The model under review builds one solid part; all positions refer to its coordinate system, in mm. Face numbers are marked on the shaded views. A direction names the side the tool comes from. Coordinates: 2 decimals unless noted, no trailing zeros. Write each loop counter-clockwise with the first axis right and the second up, starting at its lowest first coordinate (ties: lowest second). Pieces come first, ordered by that corner, then holes. Notation, with made-up numbers: M 74.5,71 L 98.5,71 A9 ccw 98.5,88 Z; hole C 36,63.5 d11. An arc over 180 degrees is marked long. Answer as a JSON object with one key per item and string values.
```python
from build123d import *

# Parameters (mm, degrees)
SKETCH2_W           = 56.399999976
SKETCH2_H           = 56.399999976
SKETCH2_R           = 15.8877
SKETCH2_R_2         = 2.499999953
BOSS_EXTRUDE1_DEPTH = 6.35
SKETCH2_4_R         = 19.05
SKETCH2_4_R_2       = 15.8877
CUT_EXTRUDE2_DEPTH  = 1.600000102
SKETCH3_R           = 25.4
SKETCH3_R_2         = 19.05
BOSS_EXTRUDE2_DEPTH = 47.625
SKETCH4_R           = 2.5
SKETCH4_R_2         = 7.62
BOSS_EXTRUDE3_DEPTH = 6.35
FILLET1_R           = 2.54


with BuildPart() as part:
    # Sketch2 → Boss-Extrude1 (new body)
    with BuildSketch(Plane(origin=(0, 0, 0), x_dir=(1, 0, 0), z_dir=(0, 1, 0))):
        Rectangle(SKETCH2_W, SKETCH2_H)
        with Locations(Location((0, 0, 0), (0, 0, 270))):
            Circle(SKETCH2_R, mode=Mode.SUBTRACT)
        with Locations(Location((23.569999977, 23.569999977, 0), (0, 0, 270))):
            Circle(SKETCH2_R_2, mode=Mode.SUBTRACT)
        with Locations(Location((23.569999977, -23.569999977, 0), (0, 0, 270))):
            Circle(SKETCH2_R_2, mode=Mode.SUBTRACT)
        with Locations(Location((-23.569999977, -23.569999977, 0), (0, 0, 270))):
            Circle(SKETCH2_R_2, mode=Mode.SUBTRACT)
        with Locations(Location((-23.569999977, 23.569999977, 0), (0, 0, 270))):
            Circle(SKETCH2_R_2, mode=Mode.SUBTRACT)
    extrude(amount=-BOSS_EXTRUDE1_DEPTH)

    # Sketch2<4> → Cut-Extrude2 (cut)
    with BuildSketch(Plane(origin=(0, 0, 0), x_dir=(1, 0, 0), z_dir=(0, 1, 0))):
        with Locations(Location((0, 0, 0), (0, 0, 270))):
            Circle(SKETCH2_4_R)
        with Locations(Location((0, 0, 0), (0, 0, 270))):
            Circle(SKETCH2_4_R_2, mode=Mode.SUBTRACT)
    extrude(amount=-CUT_EXTRUDE2_DEPTH, mode=Mode.SUBTRACT)

    # Sketch3 → Boss-Extrude2 (add)
    with BuildSketch(Plane.XZ.offset(6.35)):
        with Locations(Location((0, 0, 0), (0, 0, 270))):
            Circle(SKETCH3_R)
        with Locations(Location((0, 0, 0), (0, 0, 90))):
            Circle(SKETCH3_R_2, mode=Mode.SUBTRACT)
    extrude(amount=BOSS_EXTRUDE2_DEPTH)

    # Sketch4 → Boss-Extrude3 (add)
    with BuildSketch(Plane.XZ.offset(53.975)):
        with BuildLine():
            Line((38.1, -14.999999972), (38.1, 14.999999972))
            Line((38.1, 14.999999972), (20.497804781, 14.999999972))
            ThreePointArc((20.497804781, 14.999999972), (0, 25.4), (-20.497804781, 14.999999972))
            Line((-20.497804781, 14.999999972), (-38.1, 14.999999972))
            Line((-38.1, 14.999999972), (-38.1, -14.999999972))
            Line((-38.1, -14.999999972), (-20.497804781, -14.999999972))
            ThreePointArc((-20.497804781, -14.999999972), (0, -25.4), (20.497804781, -14.999999972))
            Line((20.497804781, -14.999999972), (38.1, -14.999999972))
        make_face()
        with Locations(Location((-33.655, -10.554999972, 0), (0, 0, 270))):
            Circle(SKETCH4_R, mode=Mode.SUBTRACT)
        with Locations(Location((0, 0, 0), (0, 0, 270))):
            Circle(SKETCH4_R_2, mode=Mode.SUBTRACT)
        with Locations(Location((-33.655, 10.554999972, 0), (0, 0, 270))):
            Circle(SKETCH4_R, mode=Mode.SUBTRACT)
        with Locations(Location((33.655, -10.554999972, 0), (0, 0, 270))):
            Circle(SKETCH4_R, mode=Mode.SUBTRACT)
        with Locations(Location((33.655, 10.554999972, 0), (0, 0, 270))):
            Circle(SKETCH4_R, mode=Mode.SUBTRACT)
    extrude(amount=BOSS_EXTRUDE3_DEPTH)

    # Fillet1
    # the kernel refuses this fillet: 2.54 mm, written as the material it adds along each edge
    with BuildSketch(Plane(origin=(20.497804781, -53.975, 14.999999972), x_dir=(-0.6093303633188096, 0, 0.7929164573508154), z_dir=(0, -1, 0)), Plane(origin=(-20.497804781, -53.975, -14.999999972), x_dir=(0.609330363318784, 0, -0.7929164573508352), z_dir=(0, -1, 0))) as fillet1_piece_1:
        with BuildLine():
            CenterArc((1.251994792, -2.539300218), FILLET1_R, 91.344968241, 51.113932151)
            Line((-0.762013009, -0.991601095), (0, 0))
            ThreePointArc((0, 0), (0.596187996, -0.006997817), (1.192375993, 0))
        make_face()
    extrude(amount=6.35)
    with BuildSketch(Plane(origin=(-20.497804781, -53.975, 14.999999972), x_dir=(0.6093303633187793, 0, 0.7929164573508387), z_dir=(0, -1, 0)), Plane(origin=(20.497804781, -53.975, -14.999999972), x_dir=(-0.609330363318815, 0, -0.7929164573508114), z_dir=(0, -1, 0))) as fillet1_piece_2:
        with BuildLine():
            CenterArc((1.251994792, 2.539300218), FILLET1_R, 217.541099608, 51.113932151)
            Line((-0.762013009, 0.991601095), (0, 0))
            ThreePointArc((0, 0), (0.596187996, 0.006997817), (1.192375993, 0))
        make_face()
    extrude(amount=6.35)
    # the kernel refuses this fillet: 2.54 mm, written as the material it takes off along each edge
    with BuildSketch(Plane(origin=(-28.199999988, 6.35, -28.199999988), x_dir=(0, 0, 1), z_dir=(0, -1, 0)), Plane(origin=(-28.199999988, 6.35, 28.199999988), x_dir=(1, 0, 0), z_dir=(0, -1, 0)), Plane(origin=(38.1, -47.625, -14.999999972), x_dir=(-1, 0, 0), z_dir=(0, -1, 0)), Plane(origin=(38.1, -47.625, 14.999999972), x_dir=(0, 0, -1), z_dir=(0, -1, 0))) as fillet1_2_piece_1:
        with BuildLine():
            CenterArc((FILLET1_R, -FILLET1_R), FILLET1_R, 90, 90)
            Line((0, -FILLET1_R), (0, 0))
            Line((0, 0), (FILLET1_R, 0))
        make_face()
    extrude(amount=19.05, mode=Mode.SUBTRACT)
    with BuildSketch(Plane(origin=(28.199999988, 6.35, -28.199999988), x_dir=(0, 0, 1), z_dir=(0, -1, 0)), Plane(origin=(28.199999988, 6.35, 28.199999988), x_dir=(-1, 0, 0), z_dir=(0, -1, 0)), Plane(origin=(-38.1, -47.625, 14.999999972), x_dir=(0, 0, -1), z_dir=(0, -1, 0)), Plane(origin=(-38.1, -47.625, -14.999999972), x_dir=(1, 0, 0), z_dir=(0, -1, 0))) as fillet1_2_piece_2:
        with BuildLine():
            CenterArc((FILLET1_R, FILLET1_R), FILLET1_R, 180, 90)
            Line((0, FILLET1_R), (0, 0))
            Line((0, 0), (FILLET1_R, 0))
        make_face()
    extrude(amount=19.05, mode=Mode.SUBTRACT)


solid = part.part
```
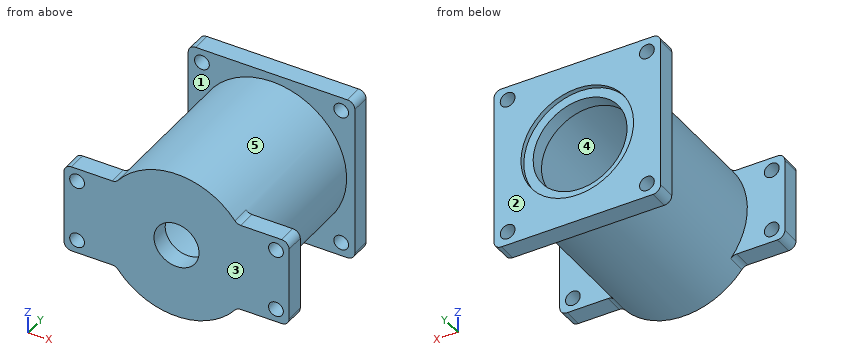
(1) Wall thickness on line 1 along X through (y, z) = (-3, 23.57); line 2 along X through (y, z) = (-55.5, 0); line 3 along X through (y, z) = (-26, 0): over which ranges is each line inside the solid? List them lowest first. Write a range as from..to.
Results list:
{"line 1": "-28.2..-26.07, -21.07..21.07, 26.07..28.2", "line 2": "-38.1..-7.62, 7.62..38.1", "line 3": "-25.4..-19.05, 19.05..25.4"}
(2) Draft analysis for pull direction X (two halves, no side actions). For the marked faces 3, 4 and 5, state which applies: released by +X, released by -X, zero draft, split by the parting line, or undercut.
Results list:
{"face 3": "zero draft", "face 4": "undercut", "face 5": "split by the parting line"}
(3) Add section D-D on x = -23.57. Give the boundary of the cut face in (y, z) (3 decimals).
Results list:
{"outline": "M -60.325,-15 L -53.975,-15 L -53.975,-9.467 L -6.35,-9.467 L -6.35,-21.07 L 0,-21.07 L 0,21.07 L -6.35,21.07 L -6.35,9.467 L -53.975,9.467 L -53.975,15 L -60.325,15 Z; M -6.35,-28.2 L 0,-28.2 L 0,-26.07 L -6.35,-26.07 Z; M -6.35,26.07 L 0,26.07 L 0,28.2 L -6.35,28.2 Z"}
(4) Add section C-C on z = 23.57. Give the boundary of the cut face in (x, y) (3 decimals), and give its area (3 significant figures).
Results list:
{"outline": "M -28.2,-6.35 L -26.07,-6.35 L -26.07,0 L -28.2,0 Z; M -21.07,-6.35 L -9.467,-6.35 L -9.467,-60.325 L 9.467,-60.325 L 9.467,-6.35 L 21.07,-6.35 L 21.07,0 L -21.07,0 Z; M 26.07,-6.35 L 28.2,-6.35 L 28.2,0 L 26.07,0 Z", "area": "1,320 mm²"}
(5) For the marked faces 1 and 2, list the 3-axis set-ups (+Z, -Z, +X, -X, +Y, -Y) from which the entire face can be reached by the end or side of a thin tool; tool diameter is ignored.
Results list:
{"face 1": "none", "face 2": "+Z, -Z, +X, -X, +Y"}
(6) Add section B-B on z = 0. Give the boundary of the cut face in (x, y) (3 decimals).
Results list:
{"outline": "M -38.1,-60.325 L -7.62,-60.325 L -7.62,-53.975 L -19.05,-53.975 L -19.05,-6.35 L -15.888,-6.35 L -15.888,-1.6 L -19.05,-1.6 L -19.05,0 L -28.2,0 L -28.2,-6.35 L -25.4,-6.35 L -25.4,-53.975 L -38.1,-53.975 Z; M 7.62,-60.325 L 38.1,-60.325 L 38.1,-53.975 L 25.4,-53.975 L 25.4,-6.35 L 28.2,-6.35 L 28.2,0 L 19.05,0 L 19.05,-1.6 L 15.888,-1.6 L 15.888,-6.35 L 19.05,-6.35 L 19.05,-53.975 L 7.62,-53.975 Z"}
(7) Add section A-A on x = 0. Give the boundary of the cut face in (y, z) (3 decimals).
Results list:
{"outline": "M -60.325,-25.4 L -6.35,-25.4 L -6.35,-28.2 L 0,-28.2 L 0,-19.05 L -1.6,-19.05 L -1.6,-15.888 L -6.35,-15.888 L -6.35,-19.05 L -53.975,-19.05 L -53.975,-7.62 L -60.325,-7.62 Z; M -60.325,7.62 L -53.975,7.62 L -53.975,19.05 L -6.35,19.05 L -6.35,15.888 L -1.6,15.888 L -1.6,19.05 L 0,19.05 L 0,28.2 L -6.35,28.2 L -6.35,25.4 L -60.325,25.4 Z"}
(8) For pin 1 Ø17.5 at (x, z) = (0, 0) entering from +Y (3 decimals); pin 2 Ø7 at (x, y) = (-27.5, -57.5) entering from -Z; pin 3 Ø2 at (y, z) = (-47.5, -11) entering from -X, all flat-tipped, find the tip position at first contact; note any pin that passes through.
Results list:
{"pin 1": "y = -53.975", "pin 2": "z = -15", "pin 3": "x = -23.35"}
